Input: dimensioned drawing with shaded views. Units: mm. Origin: part minimum x, y, z. A direction names the side the tool comes from. Give positions to 0.01 mm unless a question says otherwise; leave off trailing zeros. Order: outer loops, then holes, each group sorted by start corner. A loop starts at its lowest first (then second) coordinate and runs counter-clockwise, first axis right, second up. Notation, with made-up numbers: M -19.5,6 L -13.5,6 A25 ccw -13.5,38 Z; hole C -16,68.5 d1. An arc over 180 degrees is marked long. Answer in a Markdown table with one row per item. Add a question column.
(1) Pin query (flat end, axial travel): P1, Ø20.5, axis at x = 25.4, z = 50.8, coming from the -Y side; P2, Ø5, axis at x = 96, y = 36.5, coming from the +Z side (1 decimal); P3, Ø8, axis at y = 43, z = 19.5, coming from the -X side; P4, Ø12.5, axis at x = 94.5, y = 15, coming from the +Z side. Return the tip coordinate at first contact, or that it passes through.
(2) Section query A-A, the plane y = 15. Return loops of the section in (x, z), plus the area to 3 significant figures.
(3) Section query C-C, the plane z = 42.5. Return loops of the section in (x, y), plus the area to 3 significant figures.
(4) Material intervals for line 1 along Z through (x, y) = (25, 22); line 2 along X through (y, z) = (17, 50) (1 decimal); line 3 along Z through (x, y) = (112, 18.5), sorted ascending.
(5) Set-up query: the marked faces 1, 2 and 3. Return all of +Z, -Z, +X, -X, +Y, -Y with unobstructed straight access to the full face (end or side cutting, diameter ignored); none if empty.
(6) Mould query, pull axis X, two halves, no side actions, for the marked faces 4, 5, 6 and 7. Classes: pulls with the +X half, pulls with the -X half, needs draft (parallel to the pull), parting line crosses it, or undercut.
(7) Section query B-B, the plane x = 25.4. Return loops of the section in (y, z), plus the area to 3 significant figures.
(8) Section query D-D, the plane x = 80. Return loops of the section in (y, z), plus the area to 3 significant figures.
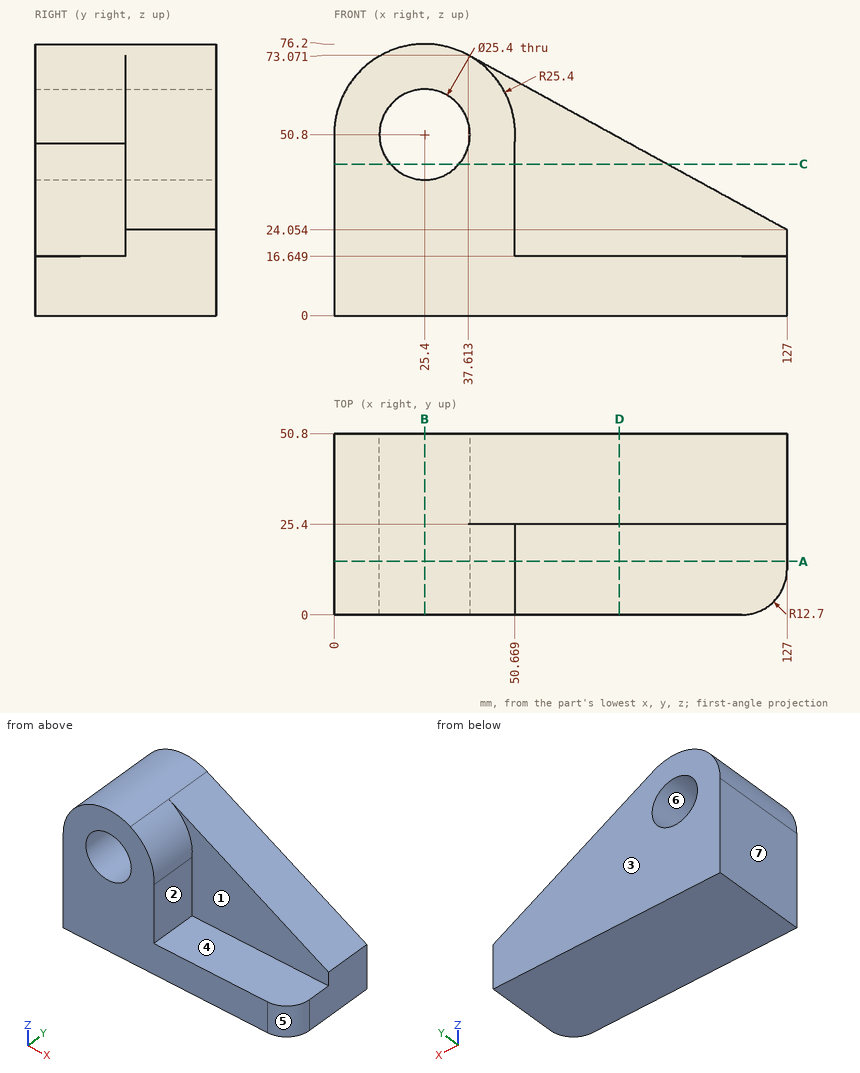
Values follow:
| question | item | result |
|---|---|---|
| 1 | P1 | passes through |
| 1 | P2 | stops at z = 42.4 |
| 1 | P3 | stops at x = 0 |
| 1 | P4 | stops at z = 16.65 |
| 2 | outline | M 0,0 L 127,0 L 127,16.65 L 50.67,16.65 L 50.67,48.22 A25.4 ccw 37.61,73.07 A25.4 ccw 0,50.8 Z; hole C 25.4,50.8 d25.4 |
| 2 | area | 4,350 mm² |
| 3 | outline | M 0,0 L 15.79,0 L 15.79,50.8 L 0,50.8 Z; M 35.01,0 L 50.67,0 L 50.67,25.4 L 93.36,25.4 L 93.36,50.8 L 35.01,50.8 Z |
| 3 | area | 2,680 mm² |
| 4 | line 1 | z = 0 to 38.11, 63.49 to 76.2 |
| 4 | line 2 | x = 0 to 12.7, 38.1 to 50.8 |
| 4 | line 3 | z = 0 to 16.65 |
| 5 | face 1 | +Z, +X, -Y |
| 5 | face 2 | +X, -Y |
| 5 | face 3 | +Z, -Z, +X, -X, +Y |
| 6 | face 4 | needs draft |
| 6 | face 5 | pulls with the +X half |
| 6 | face 6 | undercut |
| 6 | face 7 | pulls with the -X half |
| 7 | outline | M 0,0 L 50.8,0 L 50.8,38.1 L 0,38.1 Z; M 0,63.5 L 50.8,63.5 L 50.8,76.2 L 0,76.2 Z |
| 7 | area | 2,580 mm² |
| 8 | outline | M 0,0 L 50.8,0 L 50.8,49.83 L 25.4,49.83 L 25.4,16.65 L 0,16.65 Z |
| 8 | area | 1,690 mm² |
